Input: part model. Units: mm. Frame: model coordinates. A direction names the side the tool comes from. Give positions to 0.01 mm unless a question says otherwise; leave off trailing zeros. Write each loop counter-clockwise with the first axis right and the second up, starting at its lowest first coordinate (ties: lowest second). Pieces come first, ordered by that corner, then holes. Notation, with made-up numbers: (35, -39) -> (91, -39) arc R13 ccw to (91, -17) -> close; hole circle Ø4 at (7.25, 14). An arc over 180 degrees is marked (long way). Return JSON: item names as keys, results as strings. Group by question number.
Item 1: Section C-C, the plane z = -1.75. Return loops of the section in (x, y), then the cut area to 3 significant figures.
Item 2: Pin query (flat end, axial travel): P1, Ø4, axis at x = 13.5, z = -4.5, coming from the -Y side; P2, Ø3.5, axis at x = 19, y = 2, coming from the +Z side; P3, Ø3, axis at x = 15, z = -4.5, coming from the -Y side. Return the tip coordinate at first contact, or that it passes through.
Item 3: Section D-D, the plane x = 27.5. Return loops of the section in (y, z), then the cut area to 3 significant figures.
Item 4: Section A-A, the plane y = -2.75. Return loops of the section in (x, z), then the cut area to 3 significant figures.
Item 5: Line query: line 1 (X direction, y = 5.25, z = 0.5); line 2 (Z direction, x = 27, y = 2.5); line 3 (Z direction, x = 16.5, y = 0). Output: solid intervals per line, ascending. Write a range as [from, to].
Item 6: Mould query, pull axis Y, two halves, no side actions, for faces 4 (the face through (28, -6, 0)), 5 (the face through (15.2, -3.2, -2.4)), 6 (the face through (30, -1.4, 4.1)). Classes: released by +Y, released by -Y, zero draft, split by the parting line, or undercut.
Item 7: Set-up query: faces 1 (the face through (14.85, -3.85, -4.6)), 2 (the face through (4, -5, -5)), 3 (the face through (15, 2, -4)). Return all of +Z, -Z, +X, -X, +Y, -Y with unobstructed straight access to the full face (end or side cutting, diameter ignored); none if empty.
from build123d import *

# Parameters (mm, degrees)
F0_R     = 6
F1_DEPTH = 30
F2_R     = 4
F3_DEPTH = 30.001
F6_DEPTH = 22
F7_W     = 12
F7_H     = 12
F7_R     = 4
F9_DEPTH = 4


# Not quite as in the source:
# - a pattern or mirror of a feature is missing from the dataset's text; its kind, count and spacing are read off the source's solid


with BuildPart() as f1:
    # F0 (on Right) → F1 (new body)
    with BuildSketch(Plane.YZ):
        Circle(F0_R)
    extrude(amount=F1_DEPTH)

    # F2 (on face) → F3 (cut, through all)
    with BuildSketch(Plane.YZ.offset(30)):
        Circle(F2_R)
    extrude(amount=-F3_DEPTH, mode=Mode.SUBTRACT)

    # F5 (on offset) → F6 (cut)
    with BuildSketch(Plane.YZ.offset(26)):
        with BuildLine():
            Line((0, 0), (0, -4))
            Line((0, -4), (8, -4))
            Line((8, -4), (8.9776590466, 9.4645246863))
            Line((8.9776590466, 9.4645246863), (-7.7182371169, 9.4645246863))
            Line((-7.7182371169, 9.4645246863), (-7.7182371169, 3.5))
            Line((-7.7182371169, 3.5), (-4.5, 3.5))
            ThreePointArc((-4.5, 3.5), (-3.7928932188, 3.2071067812), (-3.5, 2.5))
            Line((-3.5, 2.5), (-3.5, 0))
            Line((-3.5, 0), (0, 0))
        make_face()
    extrude(amount=-F6_DEPTH, mode=Mode.SUBTRACT)

    # F7 (on face) → F9 (join)
    with BuildSketch(Plane.YZ.offset(30)):
        Rectangle(F7_W, F7_H)
        Circle(F7_R, mode=Mode.SUBTRACT)
    f9 = extrude(amount=-F9_DEPTH)

    # F9_copies: F9 across plane
    add(f9.mirror(Plane(origin=(15, 0, 0), x_dir=(0, 0, -1), z_dir=(-1, 0, 0))))


solid = f1.part
Answer below:
{
 "1": {"outline": "(0, -6) -> (4, -6) -> (4, -5.74) -> (26, -5.74) -> (26, -6) -> (30, -6) -> (30, -3.6) -> (0, -3.6) -> close; (0, 3.6) -> (4, 3.6) -> (4, 6) -> (0, 6) -> close; (26, 3.6) -> (30, 3.6) -> (30, 6) -> (26, 6) -> close", "area": "85.6 mm2"},
 "2": {"P1": "stops at y = -5.45", "P2": "stops at z = -4", "P3": "stops at y = -5.2"},
 "3": {"outline": "(-6, -6) -> (6, -6) -> (6, 6) -> (-6, 6) -> close; hole circle Ø8 at (0, 0)", "area": "93.7 mm2"},
 "4": {"outline": "(0, -6) -> (4, -6) -> (4, -5.33) -> (26, -5.33) -> (26, -6) -> (30, -6) -> (30, -2.9) -> (0, -2.9) -> close; (0, 2.9) -> (4, 2.9) -> (4, 6) -> (0, 6) -> close; (26, 2.9) -> (30, 2.9) -> (30, 6) -> (26, 6) -> close", "area": "103 mm2"},
 "5": {"line 1": "x = [0, 4], [26, 30]", "line 2": "z = [-6, -3.12], [3.12, 6]", "line 3": "z = [-6, -4]"},
 "6": {"face 4": "released by -Y", "face 5": "undercut", "face 6": "zero draft"},
 "7": {"face 1": "none", "face 2": "-Z, -Y", "face 3": "+Z, +Y"}
}
